CAD build for the part. Positions are in the model's coordinates, mm. Face numbers are marked on the shaded views. Round coordinates to 2 decimals unless told otherwise and drop trailing zeros. Write each loop counter-clockwise with the first axis right and the second up, starting at its lowest first coordinate (ties: lowest second). Pieces come first, ordered by that corner, then holes. Notation, with made-up numbers: (32, 22) - (58, 22) arc R27 cw to (58, 51) - close; hole circle Ø6 at (-0.75, 76.5). An arc over 180 degrees is marked (long way). Put each result on its own line as item: value. Start each with the question number.
Item 1: Drill centre lines: line 1 (X direction, y = 0, z = 14.55); line 2 (Y direction, x = 0, z = 15.2); line 3 (Y direction, x = 23, z = 14.85). Where is each one in solid material? Low to high. Write a range as from..to.
Item 2: Mould opens along X. For the marked faces 1, 2, 3 and 4 say: released by +X, released by -X, zero draft, split by the parting line, or undercut.
Item 3: Cut at D-D (y = 6.5). Give the cut face in (x, z).
Item 4: Cut at C-C (x = 5.5). Give the cut face in (y, z).
Item 5: Cut at A-A (y = 0). Give the cut face in (x, z).
Item 6: Pin check, flat tip, straight feed: pin 1 Ø1.8 at (x, y) = (23, 0) entering from -Z. Stop position of the tip, or through.
Item 7: Cut at B-B (z = 15.65). Give the cut face in (x, y), and give its area (3 significant figures).
```python
from build123d import *

# Parameters (mm, degrees)
SKETCH1_R           = 1.5
BOSS_EXTRUDE1_DEPTH = 16
SKETCH3_W           = 48.560524615
SKETCH3_H           = 12
CUT_EXTRUDE1_DEPTH  = 38.566607513
SKETCH4_W           = 40.711523195
SKETCH4_H           = 24.869533466
CUT_EXTRUDE2_DEPTH  = 10


with BuildPart() as part:
    # Sketch1 → Boss-Extrude1 (new body)
    with BuildSketch(Plane.XY):
        with BuildLine():
            ThreePointArc((23, 7.5), (30.5, 0), (23, -7.5))
            Line((23, -7.5), (0, -5))
            ThreePointArc((0, -5), (-5, 0), (0, 5))
            Line((0, 5), (23, 7.5))
        make_face()
        with Locations((23, 0)):
            Circle(SKETCH1_R, mode=Mode.SUBTRACT)
        Circle(SKETCH1_R, mode=Mode.SUBTRACT)
    extrude(amount=BOSS_EXTRUDE1_DEPTH)

    # Sketch3 → Cut-Extrude1 (cut, through all)
    with BuildSketch(Plane(origin=(0, 7.5, 0), x_dir=(1, 0, 0), z_dir=(0, 1, 0))):
        with Locations((17.305581285, -8)):
            Rectangle(SKETCH3_W, SKETCH3_H)
    extrude(amount=-CUT_EXTRUDE1_DEPTH, mode=Mode.SUBTRACT)


with BuildPart() as cut_extrude1_piece_1:
    # of the separate pieces the step leaves, piece 1, a body of its own (cut_extrude1_pieces)
    add(part.part.solids().sort_by_distance((0, 5, 0))[0])

    # Sketch4 → Cut-Extrude2 (cut)
    with BuildSketch(Plane(origin=(0, 0, 0), x_dir=(-1, 0, 0), z_dir=(0, 0, -1))):
        with Locations((-12.191435823, 3.299568453)):
            Rectangle(SKETCH4_W, SKETCH4_H)
    extrude(amount=-CUT_EXTRUDE2_DEPTH, mode=Mode.SUBTRACT)


with BuildPart() as cut_extrude1_piece_2:
    # of the separate pieces the step leaves, piece 2, a body of its own (cut_extrude1_pieces)
    add(part.part.solids().sort_by_distance((0, 5, 14))[0])


solid = cut_extrude1_piece_2.part
```
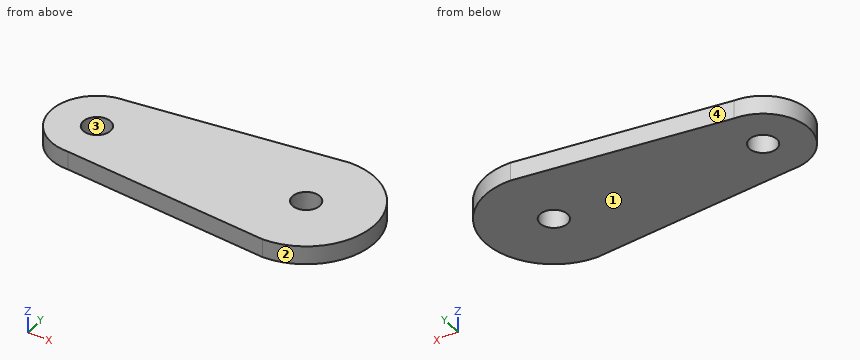
Output values:
1. line 1: -5..-1.5, 1.5..21.5, 24.5..30.5
1. line 2: -5..-1.5, 1.5..5
1. line 3: -7.5..-1.5, 1.5..7.5
2. face 1: zero draft
2. face 2: released by +X
2. face 3: undercut
2. face 4: released by -X
3. outline: (13.8, 14) - (26.74, 14) - (26.74, 16) - (13.8, 16) - close
4. outline: (-5.6, 14) - (5.6, 14) - (5.6, 16) - (-5.6, 16) - close
5. outline: (-5, 14) - (-1.5, 14) - (-1.5, 16) - (-5, 16) - close; (1.5, 14) - (21.5, 14) - (21.5, 16) - (1.5, 16) - close; (24.5, 14) - (30.5, 14) - (30.5, 16) - (24.5, 16) - close
6. pin 1: through
7. outline: (0, -5) - (23, -7.5) arc R7.5 ccw to (23, 7.5) - (0, 5) arc R5 ccw to start; hole circle Ø3 at (0, 0); hole circle Ø3 at (23, 0)
7. area: 401 mm2
